Verification items for the finished model (mm, model axes). A direction names the side the tool comes from. Give positions to 0.01 mm unless a question says otherwise; leave off trailing zeros. Write each loop counter-clockwise with the first axis right and the second up, starting at its lowest first coordinate (ties: lowest second). Pieces come first, ordered by that corner, then holes. Notation, with made-up numbers: M 49.5,-25 L 74.5,-25 A20 ccw 74.5,12 Z; hole C 43,17.25 d6. An arc over 180 degrees is marked long. Answer as a JSON object with one key per item and string values.
```python
from build123d import *

# Parameters (mm, degrees)
F1_DEPTH = 20


with BuildPart() as f1:
    # F0 (on Right) → F1 (new body)
    with BuildSketch(Plane.YZ):
        with BuildLine():
            Line((-65.767472, 6), (-83, 6))
            ThreePointArc((-83, 6), (-84.414214, 5.414214), (-85, 4))
            Line((-85, 4), (-85, 2))
            ThreePointArc((-85, 2), (-84.414214, 0.585786), (-83, 0))
            Line((-83, 0), (-65.767472, 0))
            ThreePointArc((-65.767472, 0), (-65.050944, 0.132759), (-64.429543, 0.513412))
            Line((-64.429543, 0.513412), (-45.570457, 17.486588))
            ThreePointArc((-45.570457, 17.486588), (-44.949056, 17.867241), (-44.232528, 18))
            Line((-44.232528, 18), (0, 18))
            Line((0, 18), (0, 24))
            Line((0, 24), (-44.232528, 24))
            ThreePointArc((-44.232528, 24), (-44.949056, 23.867241), (-45.570457, 23.486588))
            Line((-45.570457, 23.486588), (-64.429543, 6.513412))
            ThreePointArc((-64.429543, 6.513412), (-65.050944, 6.132759), (-65.767472, 6))
        make_face()
        with BuildLine():
            Line((44.232528, 24), (0, 24))
            Line((0, 24), (0, 18))
            Line((0, 18), (44.232528, 18))
            ThreePointArc((44.232528, 18), (44.949056, 17.867241), (45.570457, 17.486588))
            Line((45.570457, 17.486588), (64.429543, 0.513412))
            ThreePointArc((64.429543, 0.513412), (65.050944, 0.132759), (65.767472, 0))
            Line((65.767472, 0), (83, 0))
            ThreePointArc((83, 0), (84.414214, 0.585786), (85, 2))
            Line((85, 2), (85, 4))
            ThreePointArc((85, 4), (84.414214, 5.414214), (83, 6))
            Line((83, 6), (65.767472, 6))
            ThreePointArc((65.767472, 6), (65.050944, 6.132759), (64.429543, 6.513412))
            Line((64.429543, 6.513412), (45.570457, 23.486588))
            ThreePointArc((45.570457, 23.486588), (44.949056, 23.867241), (44.232528, 24))
        make_face()
    extrude(amount=F1_DEPTH)


solid = f1.part
```
1) Section check B-B on z = 16. Record the boundary of the cut face in (x, y), and give its area (3 significant figures).
Completed:
{"outline": "M 0,-53.89 L 20,-53.89 L 20,-47.22 L 0,-47.22 Z; M 0,47.22 L 20,47.22 L 20,53.89 L 0,53.89 Z", "area": "267 mm2"}
2) Section check A-A on x = 16. Record the boundary of the cut face in (y, z), and give its area (3 significant figures).
Completed:
{"outline": "M -85,2 A2 ccw -83,0 L -65.77,0 A2 ccw -64.43,0.51 L -45.57,17.49 A2 cw -44.23,18 L 44.23,18 A2 cw 45.57,17.49 L 64.43,0.51 A2 ccw 65.77,0 L 83,0 A2 ccw 85,2 L 85,4 A2 ccw 83,6 L 65.77,6 A2 cw 64.43,6.51 L 45.57,23.49 A2 ccw 44.23,24 L -44.23,24 A2 ccw -45.57,23.49 L -64.43,6.51 A2 cw -65.77,6 L -83,6 A2 ccw -85,4 Z", "area": "1,020 mm2"}
3) Section check C-C on y = -29. Record the boundary of the cut face in (x, z), and give its area (3 significant figures).
Completed:
{"outline": "M 0,18 L 20,18 L 20,24 L 0,24 Z", "area": "120 mm2"}
4) Go/stop test with flat-tipped pins: pin 1 (6 mm diameter, centred on x = 13.5, z = 16.5, fed in from +Y); pin 2 (1.5 mm diameter, centred on x = 4.5, z = 16, fed in from +Y); pin 3 (10 mm diameter, centred on x = 12, z = 20, fed in from -Y). Record where each tip stops, or that it passes through.
Completed:
{"pin 1": "stops at y = 56.67", "pin 2": "stops at y = 54.72", "pin 3": "stops at y = -55"}
5) Release check for a two-part mould opening along Y. For faces 1 (the face through (10, 74, 0)), 2 (the face through (10, -55, 9)), 3 (the face through (10, -55, 15)) record: pulls with the +Y half, pulls with the -Y half, needs draft (parallel to the pull), parting line crosses it, or undercut.
Completed:
{"face 1": "needs draft", "face 2": "undercut", "face 3": "pulls with the -Y half"}
6) Thickness scan on L1, parallel to Z at x = 10.5, y = 2; L2, parallel to Y at x = 17.75, z = 2.25; L3, parallel to Y at x = 16.25, z = 13.5. Record the ranges inside material, lowest first.
Completed:
{"L1": "z = 18 to 24", "L2": "y = -85 to -62.5, 62.5 to 85", "L3": "y = -56.67 to -50, 50 to 56.67"}
7) Access from +Z, -Z, +X, -X, +Y, -Y to the whole of each face (thin tool, end or side, straight path). Record for faces 4 (the face through (10, -74, 6)), 5 (the face through (10, -1, 18)), 6 (the face through (0, -0.4, 18.3)), 7 (the face through (10, 75, 6)).
Completed:
{"face 4": "+Z, +X, -X, -Y", "face 5": "-Z, +X, -X", "face 6": "+Z, -Z, -X, +Y, -Y", "face 7": "+Z, +X, -X, +Y"}
